```python
from build123d import *

# Parameters (mm, degrees)
IZIM1_R                          = 6
Y_KSEKLIK_EKSTR_ZYON1_DEPTH      = 21
IZIM2_R                          = 6
Y_KSEKLIK_EKSTR_ZYON2_DEPTH      = 21
IZIM3_R                          = 6
Y_KSEKLIK_EKSTR_ZYON3_DEPTH      = 287
Y_KSEKLIK_EKSTR_ZYON3_DEPTH_BACK = 287
Y_KSEKLIK_EKSTR_ZYON4_DEPTH      = 42


with BuildPart() as part:
    # izim1 → Y_kseklik-Ekstr_zyon1 (new body, symmetric)
    with BuildSketch(Plane(origin=(0, 0, 0), x_dir=(0, 0, -1), z_dir=(1, 0, 0))):
        with BuildLine():
            Line((-35, 18), (35, 18))
            ThreePointArc((35, 18), (53, 0), (35, -18))
            Line((35, -18), (-35, -18))
            ThreePointArc((-35, -18), (-53, 0), (-35, 18))
        make_face()
        with Locations((-35, 0)):
            Circle(IZIM1_R, mode=Mode.SUBTRACT)
        with Locations((35, 0)):
            Circle(IZIM1_R, mode=Mode.SUBTRACT)
    extrude(amount=Y_KSEKLIK_EKSTR_ZYON1_DEPTH, both=True)


with BuildPart() as body_2:
    # izim2 → Y_kseklik-Ekstr_zyon2 (new body, symmetric)
    with BuildSketch(Plane.ZY.offset(261)):
        with BuildLine():
            Line((15, 73), (-15, 73))
            Line((-15, 73), (-35, 18))
            ThreePointArc((-35, 18), (-53, 0), (-35, -18))
            Line((-35, -18), (35, -18))
            ThreePointArc((35, -18), (53, 0), (35, 18))
            Line((35, 18), (15, 73))
        make_face()
        with Locations((35, 0)):
            Circle(IZIM2_R, mode=Mode.SUBTRACT)
        with Locations((-35, 0)):
            Circle(IZIM2_R, mode=Mode.SUBTRACT)
    extrude(amount=Y_KSEKLIK_EKSTR_ZYON2_DEPTH, both=True)


with BuildPart() as body_3:
    # Aynalama1: mirrored copy
    add(part.part.mirror(Plane.ZY.offset(261)))


with BuildPart() as part_1:
    add(part.part)

    add(body_2.part)  # Y_kseklik-Ekstr_zyon3 merges body 2

    add(body_3.part)  # Y_kseklik-Ekstr_zyon3 merges body 3
    # izim3 → Y_kseklik-Ekstr_zyon3 (add, two sides)
    with BuildSketch(Plane.ZY.offset(261)) as y_kseklik_ekstr_zyon3_sk:
        with Locations((-35, 0)):
            Circle(IZIM3_R)
        with Locations((35, 0)):
            Circle(IZIM3_R)
    extrude(amount=Y_KSEKLIK_EKSTR_ZYON3_DEPTH)
    extrude(y_kseklik_ekstr_zyon3_sk.sketch, amount=-Y_KSEKLIK_EKSTR_ZYON3_DEPTH_BACK)

    # izim4 → Y_kseklik-Ekstr_zyon4 (add)
    with BuildSketch(Plane(origin=(-240, 0, 0), x_dir=(0, 0, -1), z_dir=(1, 0, 0))):
        with BuildLine():
            ThreePointArc((-15, 73), (0, 83.446627943), (15, 73))
            Line((15, 73), (-15, 73))
        make_face()
    extrude(amount=-Y_KSEKLIK_EKSTR_ZYON4_DEPTH)


solid = part_1.part
```
Verification items for the finished model (mm, model axes). A direction names the side the tool comes from. Coordinates: 2 decimals unless noted, no trailing zeros. Order: outer loops, then holes, each group sorted by start corner. A loop starts at its lowest first (then second) coordinate and runs counter-clockwise, first axis right, second up. Notation, with made-up numbers: (14.5, 63.5) - (43.5, 63.5) arc R22 ccw to (43.5, 73.5) - close; hole circle Ø2 at (-10.5, 42.25). An arc over 180 degrees is marked (long way). Return JSON: item names as keys, results as strings.
(1) Go/stop test with flat-tipped pins: pin 1 (8 mm diameter, centred on y = 72.5, z = -3, fed in from -X); pin 2 (12.5 mm diameter, centred on x = -7.5, z = 14.5, fed in from +Y); pin 3 (12 mm diameter, centred on y = 35.5, z = 34.5, fed in from +X). Record where each tip stops, or that it passes through.
Filled sheet:
{"pin 1": "stops at x = -282", "pin 2": "stops at y = 18", "pin 3": "stops at x = -240"}
(2) Thickness scan on line 1 along X through (y, z) = (11, 4.5); line 2 along X through (y, z) = (24, -7.5); line 3 along Y through (x, z) = (-241, 36). Record the ranges inside material, lowest first.
Filled sheet:
{"line 1": "x = -543 to -501, -282 to -240, -21 to 21", "line 2": "x = -282 to -240", "line 3": "y = -17.97 to 17.97"}
(3) Section check B-B, the plane x = -367. Record the cut outline in (y, z).
Filled sheet:
{"outline": "circle Ø12 at (0, -35); circle Ø12 at (0, 35)"}
(4) Section check D-D, the plane z = -8. Record the cut outline in (x, y), and give its area (3 significant figures).
Filled sheet:
{"outline": "(-543, -18) - (-501, -18) - (-501, 18) - (-543, 18) - close; (-282, -18) - (-240, -18) - (-240, 81.3) - (-282, 81.3) - close; (-21, -18) - (21, -18) - (21, 18) - (-21, 18) - close", "area": "7,190 mm^2"}
(5) Access from +Z, -Z, +X, -X, +Y, -Y to the whole of each face (thin tool, end or side, straight path). Record for faces 1 (the cylindrical face through (23, 0, -41)), 2 (the flat face through (0, 18, 0)), 3 (the flat face through (-522, 18, 0)), 4 (the cylindrical face through (-390, 0, -41)).
Filled sheet:
{"face 1": "+X", "face 2": "+Z, -Z, +X, +Y", "face 3": "+Z, -Z, -X, +Y", "face 4": "none"}
(6) Section check A-A, the plane z = 20. Record the cut outline in (x, y), and give its area (3 significant figures).
Filled sheet:
{"outline": "(-543, -18) - (-501, -18) - (-501, 18) - (-543, 18) - close; (-282, -18) - (-240, -18) - (-240, 59.25) - (-282, 59.25) - close; (-21, -18) - (21, -18) - (21, 18) - (-21, 18) - close", "area": "6,270 mm^2"}
(7) Mould release check, pull along X, two halves, no side actions. Record for faces 5 (the flat face through (21, 0, -1)), 6 (the cylindrical face through (-389.97, -3.65, 30.24)), 7 (the flat face through (-261.29, 45.88, -24.86)): pulls with the +X half, pulls with the -X half, needs draft (parallel to the pull), parting line crosses it, or undercut.
Filled sheet:
{"face 5": "pulls with the +X half", "face 6": "undercut", "face 7": "needs draft"}
(8) Section check C-C, the plane y = 0. Give the number of separate pieces and of enclosed holes in the cut face, and give its area (3 significant figures).
Filled sheet:
{"separate pieces": "1", "enclosed holes": "2", "area": "24,100 mm^2"}
